Can you work these out from the model? Positions are in its coordinate system, mm. Face numbers are marked on the shaded views. Round coordinates to 2 decimals unless told otherwise and drop trailing zeros. Loops run counter-clockwise (first coordinate to the right, second up) from the corner with the lowest first, then second, coordinate; pieces in that order, holes last.
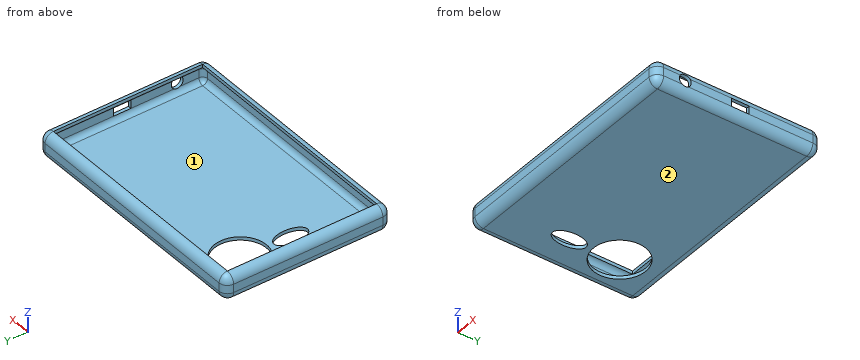
```python
from build123d import *

# Parameters (mm, degrees)
F0_W         = 150
F0_H         = 100
F1_DEPTH     = 15
F2_R         = 5
F3_T1_DEPTH  = 5
F3_S5_W      = 5
F3_S5_H      = 5
F3_T6_DEPTH  = 5
F3_S11_W     = 5
F3_S11_H     = 5
F3_T12_DEPTH = 5
F4_T         = -2
F6_R         = 15.7014328103
F7_DEPTH     = 25
F8_W         = 10.624602437
F8_H         = 5
F8_R         = 3.5673659444
F9_DEPTH     = 25


# Not quite as in the source:
# - a fillet or chamfer that OpenCascade refuses, or shapes differently, is made with other operations: its cross-section is extruded or revolved along the edge and cut away or added
# - a shell that OpenCascade refuses in one call is made with other operations: the cavity is built on its own and cut out


with BuildPart() as f1:
    # F0 (on Top) → F1 (new body)
    with BuildSketch(Plane.XY):
        Rectangle(F0_W, F0_H)
    extrude(amount=F1_DEPTH)

    # F2
    f2_edges = [f1.edges().sort_by_distance(p)[0] for p in [
        (-75, 50, 7.5),
        (-75, -50, 7.5),
        (75, -50, 7.5),
        (0, 50, 0),
        (0, -50, 0),
        (0, -50, 15),
        (-75, 0, 0),
        (-75, 0, 15),
        (75, 0, 0),
        (0, 50, 15),
        (75, 0, 15),
    ]]
    fillet(f2_edges, radius=F2_R)

    # F3: fillet of radius 5 on 1 edges, made by hand

    # F3_s2 → F3_t1 (cut)
    with BuildSketch(Plane.XY.offset(5)):
        with BuildLine():
            ThreePointArc((70, 50), (73.5355339059, 48.5355339059), (75, 45))
            Line((75, 45), (75, 50))
            Line((75, 50), (70, 50))
        make_face()
    extrude(amount=F3_T1_DEPTH, mode=Mode.SUBTRACT)


with BuildPart() as f3_tool4:
    # F3_s5 → F3_t6 (new body)
    with BuildSketch(Plane.XZ.offset(-45)):
        with Locations((72.5, 2.5)):
            Rectangle(F3_S5_W, F3_S5_H)
    extrude(amount=-F3_T6_DEPTH)

    # F3_s7 → F3_t8 (revolve, cut)
    with BuildSketch(Plane(origin=(70, 45, 5), x_dir=(-0.7071067812, 0, 0.7071067812), z_dir=(-0.7071067812, 0, -0.7071067812))):
        with BuildLine():
            ThreePointArc((0, -5), (5, 0), (0, 5))
            Line((0, 5), (0, -5))
        make_face()
    revolve(axis=Axis((70, 45, 5), (0, 1, 0)), mode=Mode.SUBTRACT)


with BuildPart() as f1_1:
    add(f1.part)

    # F3_t3: cut F3_tool4
    add(f3_tool4.part, mode=Mode.SUBTRACT)


with BuildPart() as f3_tool10:
    # F3_s11 → F3_t12 (new body)
    with BuildSketch(Plane.XZ.offset(-45)):
        with Locations((72.5, 12.5)):
            Rectangle(F3_S11_W, F3_S11_H)
    extrude(amount=-F3_T12_DEPTH)

    # F3_s13 → F3_t14 (revolve, cut)
    with BuildSketch(Plane(origin=(70, 45, 10), x_dir=(-0.7071067812, 0, -0.7071067812), z_dir=(0.7071067812, 0, -0.7071067812))):
        with BuildLine():
            ThreePointArc((0, -5), (5, 0), (0, 5))
            Line((0, 5), (0, -5))
        make_face()
    revolve(axis=Axis((70, 45, 10), (0, 1, 0)), mode=Mode.SUBTRACT)


with BuildPart() as f1_2:
    add(f1_1.part)

    # F3_t9: cut F3_tool10
    add(f3_tool10.part, mode=Mode.SUBTRACT)

    # F4: a shell. OpenCascade refuses it in one call, so the cavity is built on its own and cut out:
    # the body offset inwards by the wall thickness, plus a prism from it out through each open face.
    f4_core = offset(f1_2.part, amount=F4_T, mode=Mode.PRIVATE)
    f4_exits = [f4_core.faces().sort_by_distance(p)[0] for p in [
        (0, 0, 13),
    ]]
    add(f4_core, mode=Mode.SUBTRACT)
    extrude(f4_exits, amount=-F4_T, mode=Mode.SUBTRACT)

    # F6 (on face) → F7 (cut)
    with BuildSketch(Plane(origin=(0, 0, 0), x_dir=(1, 0, 0), z_dir=(0, 0, -1))):
        with Locations((-50.5510754883, -22.5712861866)):
            Circle(F6_R)
        with BuildLine():
            add(Edge.make_bspline(
                [(-52.28683725, 16.5926627815), (-61.667239248, 16.5926627815), (-56.977038249, 1.3871968258), (-52.28683725, -13.8182691298), (-47.596636251, 1.3871968258), (-42.906435252, 16.5926627815), (-52.28683725, 16.5926627815)],
                knots=[0, 0, 0, 2.0943951024, 2.0943951024, 4.1887902048, 4.1887902048, 6.2831853072, 6.2831853072, 6.2831853072], degree=2, weights=[1, 0.5, 1, 0.5, 1, 0.5, 1]))
        make_face()
    extrude(amount=-F7_DEPTH, mode=Mode.SUBTRACT)

    # F8 (on face) → F9 (cut)
    with BuildSketch(Plane.YZ.offset(75)):
        with Locations((1.3190158643, 7.5)):
            Rectangle(F8_W, F8_H)
        with Locations((-31.9286696613, 8.0319177359)):
            Circle(F8_R)
    extrude(amount=-F9_DEPTH, mode=Mode.SUBTRACT)


solid = f1_2.part
```
(1) Suppose I cut it at B-B (y = 17.5). Write out the boundary of the cut face in (x, z).
(2) We'd pull the mould along X, two halves only. Please class the marked faces 1 and 2: released by +X, released by -X, zero draft, split by the parting line, or undercut.
(3) For pin 1 (2 mm diameter, centred on x = 74, z = 8, fed in from -Y); pin 2 (1.6 mm diameter, centred on x = 74, y = 0, fed in from -Z); pin 3 (1 mm diameter, centred on x = 74, y = 0, fed in from +Z), each with a flat end and sliding along its axis, tell me the tip position at first contact or that it passes through.
(4) If I drill on line 1 (Y direction, x = -66, z = 7.75); line 2 (X direction, y = -27.5, z = 5); line 3 (Y direction, x = -13, z = 14), over which ranges is the centre line in solid material (lowest first)?
(5) Suppose I cut it at C-C (z = 6.5). Write out the boundary of the cut face in (x, y).
(6) Suppose I cut it at D-D (x = -20). Write out the boundary of the cut face in (y, z).
(7) Suppose I cut it at A-A (y = -21). Write out the boundary of the cut face in (x, z).
Check result:
1. outline: (-75, 5) arc R5 ccw to (-70, 0) - (-65.41, 0) - (-65.41, 2) - (-70, 2) arc R3 cw to (-73, 5) - (-73, 10) arc R3 cw to (-70, 13) - (-70, 15) arc R5 ccw to (-75, 10) - close; (-35.69, 0) - (70, 0) arc R5 ccw to (75, 5) - (75, 10) arc R5 ccw to (70, 15) - (70, 13) arc R3 cw to (73, 10) - (73, 5) arc R3 cw to (70, 2) - (-35.69, 2) - close
2. face 1: undercut
2. face 2: zero draft
3. pin 1: stops at y = -49
3. pin 2: stops at z = 1.16
3. pin 3: stops at z = 13.57
4. line 1: y = -50 to -48, 48 to 50
4. line 2: x = -75 to -73, 73 to 75
4. line 3: y = -48 to -45, 45 to 48
5. outline: (-75, -45) arc R5 ccw to (-70, -50) - (70, -50) arc R5 ccw to (75, -45) - (75, -35.15) - (73, -35.15) - (73, -45) arc R3 cw to (70, -48) - (-70, -48) arc R3 cw to (-73, -45) - (-73, 45) arc R3 cw to (-70, 48) - (70, 48) arc R3 cw to (73, 45) - (73, 6.63) - (75, 6.63) - (75, 45) arc R5 ccw to (70, 50) - (-70, 50) arc R5 ccw to (-75, 45) - close; (73, -28.71) - (75, -28.71) - (75, -3.99) - (73, -3.99) - close
6. outline: (-50, 5) arc R5 ccw to (-45, 0) - (45, 0) arc R5 ccw to (50, 5) - (50, 10) arc R5 ccw to (45, 15) - (45, 13) arc R3 cw to (48, 10) - (48, 5) arc R3 cw to (45, 2) - (-45, 2) arc R3 cw to (-48, 5) - (-48, 10) arc R3 cw to (-45, 13) - (-45, 15) arc R5 ccw to (-50, 10) - close
7. outline: (-75, 5) arc R5 ccw to (-70, 0) - (70, 0) arc R5 ccw to (75, 5) - (75, 10) arc R5 ccw to (70, 15) - (70, 13) arc R3 cw to (73, 10) - (73, 5) arc R3 cw to (70, 2) - (-70, 2) arc R3 cw to (-73, 5) - (-73, 10) arc R3 cw to (-70, 13) - (-70, 15) arc R5 ccw to (-75, 10) - close
